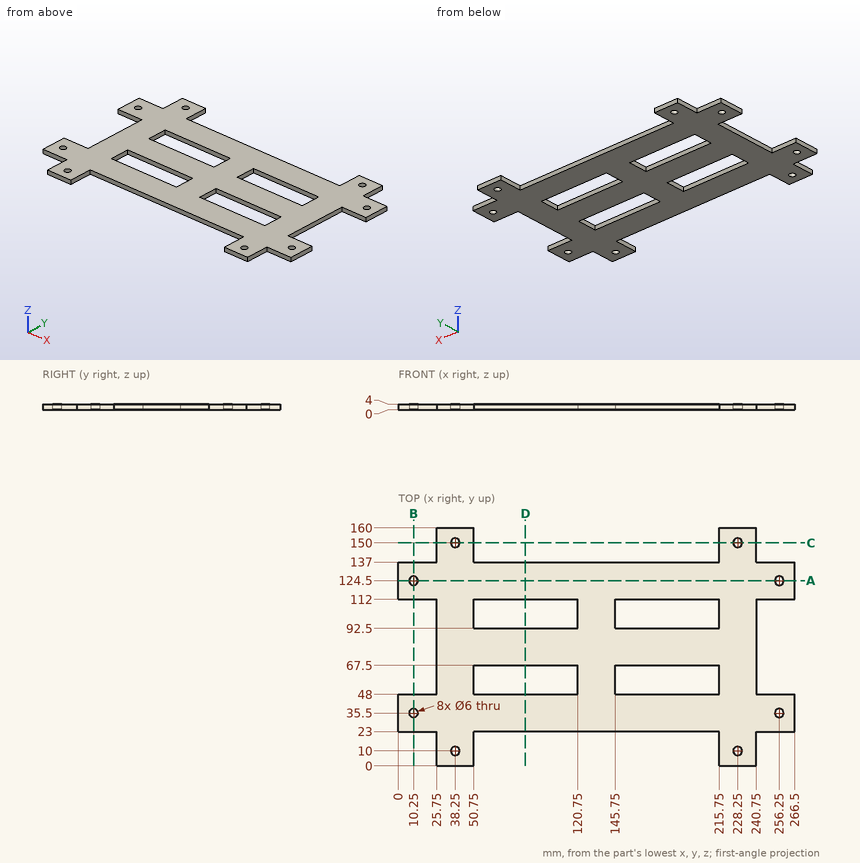
Job drawing, mm, ordinate dimensions from the low corner. One solid piece. Round coordinates to 2 decimals unless told otherwise and drop trailing zeros. Write each loop counter-clockwise with the first axis right and the second up, starting at its lowest first coordinate (ties: lowest second). Pieces come first, ordered by that corner, then holes.
1) Pin check, flat tips, straight feed: pin 1 (5 mm diameter, centred on x = 256.25, y = 35.5, fed in from -Z); pin 2 (1.2 mm diameter, centred on x = 168, z = 1, fed in from +Y); pin 3 (9.5 mm diameter, centred on x = 10.25, y = 124.5, fed in from +Z); pin 4 (2 mm diameter, centred on x = 247.5, z = 3, fed in from -Y). Stop position of each tip, or through.
2) Band-saw the part on B-B, the plane x = 10.25. List the corners of the cut face in (y, z), and give its area (3 significant figures).
3) Drill centre lines: probe 1 along X at (y, z) = (94.5, 0.7); probe 2 along X at (y, z) = (150, 2.6); probe 3 along Y at (x, z) = (228.25, 0.95). Where is each one in solid material? Low to high.
4) Band-saw the part on D-D, the plane x = 85.5. List the corners of the cut face in (y, z).
5) Band-saw the part on A-A, the plane y = 124.5. List the corners of the cut face in (x, z).
6) Band-saw the part on C-C, the plane y = 150. List the corners of the cut face in (x, z).
Ans:
1. pin 1: passes through
1. pin 2: stops at y = 137
1. pin 3: stops at z = 4
1. pin 4: stops at y = 23
2. outline: (23, 0) - (32.5, 0) - (32.5, 4) - (23, 4) - close; (38.5, 0) - (48, 0) - (48, 4) - (38.5, 4) - close; (112, 0) - (121.5, 0) - (121.5, 4) - (112, 4) - close; (127.5, 0) - (137, 0) - (137, 4) - (127.5, 4) - close
2. area: 152 mm2
3. probe 1: x = 25.75 to 50.75, 120.75 to 145.75, 215.75 to 240.75
3. probe 2: x = 25.75 to 35.25, 41.25 to 50.75, 215.75 to 225.25, 231.25 to 240.75
3. probe 3: y = 0 to 7, 13 to 147, 153 to 160
4. outline: (23, 0) - (48, 0) - (48, 4) - (23, 4) - close; (67.5, 0) - (92.5, 0) - (92.5, 4) - (67.5, 4) - close; (112, 0) - (137, 0) - (137, 4) - (112, 4) - close
5. outline: (0, 0) - (7.25, 0) - (7.25, 4) - (0, 4) - close; (13.25, 0) - (253.25, 0) - (253.25, 4) - (13.25, 4) - close; (259.25, 0) - (266.5, 0) - (266.5, 4) - (259.25, 4) - close
6. outline: (25.75, 0) - (35.25, 0) - (35.25, 4) - (25.75, 4) - close; (41.25, 0) - (50.75, 0) - (50.75, 4) - (41.25, 4) - close; (215.75, 0) - (225.25, 0) - (225.25, 4) - (215.75, 4) - close; (231.25, 0) - (240.75, 0) - (240.75, 4) - (231.25, 4) - close
